Here's how the part is built. I have some questions about the finished solid (model axes, mm). Face numbers are marked on the shaded views. A direction names the side the tool comes from. Round coordinates to 2 decimals unless told otherwise and drop trailing zeros. Loops run counter-clockwise (first coordinate to the right, second up) from the corner with the lowest first, then second, coordinate; pieces in that order, holes last. Notation, with made-up numbers: M 54,-4.75 L 98,-4.75 A25 ccw 98,27.25 Z; hole C -24,9 d10. An arc over 180 degrees is marked long. Use a Markdown table: item, result.
from build123d import *

# Parameters (mm, degrees)
F0_R     = 2.5
F1_DEPTH = 5
F2_COUNT = 18


with BuildPart() as f1:
    # F0 (on Front) → F1 (new body)
    with BuildSketch(Plane.XZ):
        with BuildLine():
            ThreePointArc((-1.0894467843, 12.4524337261), (-8.4448775952, -9.2159667101), (12.5, 0))
            ThreePointArc((12.5, 0), (9.2159667101, 8.4448775952), (1.0894467843, 12.4524337261))
            ThreePointArc((1.0894467843, 12.4524337261), (0, 12.5), (-1.0894467843, 12.4524337261))
        make_face()
        Circle(F0_R, mode=Mode.SUBTRACT)
        with BuildLine():
            ThreePointArc((-1.0894467843, 12.4524337261), (0, 12.5), (1.0894467843, 12.4524337261))
            ThreePointArc((1.0894467843, 12.4524337261), (1.0527842675, 13.7576625834), (0.6138861357, 14.9874328626))
            ThreePointArc((0.6138861357, 14.9874328626), (0, 15.0232996939), (-0.6138861357, 14.9874328626))
            ThreePointArc((-0.6138861357, 14.9874328626), (-1.0527842675, 13.7576625834), (-1.0894467843, 12.4524337261))
        make_face()
    extrude(amount=F1_DEPTH)

    # F2: F1 ×18 about axis
    f2_axis = Axis((0, 0, 0), (0, 1, 0))


with BuildPart() as f1_1:
    add(f1.part)
    for i in range(1, F2_COUNT):
        add(f1.part.rotate(f2_axis, i * 360 / F2_COUNT))


solid = f1_1.part
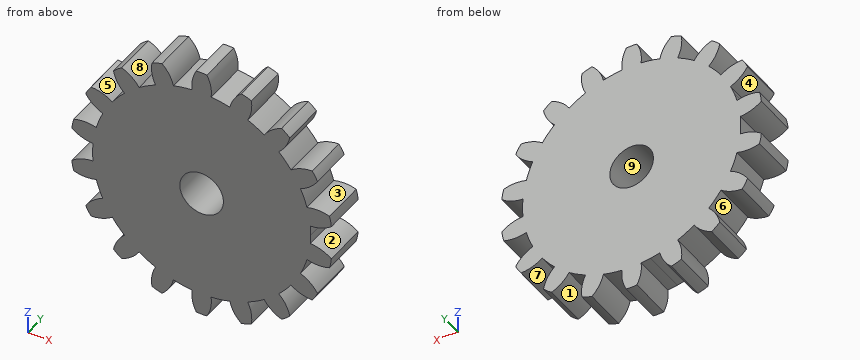
1. Which directions (+Z, -Z, +X, -X, +Y, -Y) give clear straight access to the entire face, cutting with the end or side of a thin tool? Please do the marked faces 1, 2, 3, 4 and 5.
Answer sheet:
| item | result |
|---|---|
| face 1 | -Z, +Y, -Y |
| face 2 | +X, +Y, -Y |
| face 3 | +Y, -Y |
| face 4 | -X, +Y, -Y |
| face 5 | +Z, +Y, -Y |
2. We'd pull the mould along Z, two halves only. Please class the marked faces 6, 7, 8 and 9: +Z half, -Z half, draft (parallel to the pull), parting line (faces both ways), or undercut.
Answer sheet:
| item | result |
|---|---|
| face 6 | undercut |
| face 7 | -Z half |
| face 8 | +Z half |
| face 9 | undercut |
3. I need wall thicknesses on probe 1 along Z at (x, y) = (9.5, -1.5); probe 2 along X at (y, z) = (-4.2, -13); probe 3 along X at (y, z) = (-2.7, -1). Which ranges of each line are inside material? Lowest first, please. Write a range as from..to.
Answer sheet:
| item | result |
|---|---|
| probe 1 | -11.64..-9.62, -8.12..8.12, 9.62..11.64 |
| probe 2 | -5.74..-3.56, -1.12..1.12, 3.56..5.74 |
| probe 3 | -12.46..-2.29, 2.29..12.46 |
4. Imagine slicing it at B-B, the plane z = -0.5. Write out the boundary of the cut face in (x, y).
Answer sheet:
| item | result |
|---|---|
| outline | M -12.49,-5 L -2.45,-5 L -2.45,0 L -12.49,0 Z; M 2.45,-5 L 12.49,-5 L 12.49,0 L 2.45,0 Z |
5. Imagine slicing it at C-C, the plane x = -4. Write out the boundary of the cut face in (y, z), then the cut area to 3 significant figures.
Answer sheet:
| item | result |
|---|---|
| outline | M -5,-13.71 L 0,-13.71 L 0,13.71 L -5,13.71 Z |
| area | 137 mm2 |
6. Imagine slicing it at A-A, the plane x = 0. Write out the boundary of the cut face in (y, z).
Answer sheet:
| item | result |
|---|---|
| outline | M -5,-15.02 L 0,-15.02 L 0,-2.5 L -5,-2.5 Z; M -5,2.5 L 0,2.5 L 0,15.02 L -5,15.02 Z |
7. For pin 1 Ø3 at (y, z) = (-4, -7) entering from +X, with a flat end and sliding along its axis, tell me the tip position at first contact or that it passes through.
Answer sheet:
| item | result |
|---|---|
| pin 1 | x = 13.29 |
